Source: CAD feature listing. Evaluate the final solid. Frame: model axes, mm. Give positions to 0.01 mm unless a question says otherwise; leave off trailing zeros. Loops run counter-clockwise (first coordinate to the right, second up) from the corner with the lowest first, then second, coordinate; pieces in that order, holes last. Notation, with made-up numbers: M 11.25,-11 L 24.25,-11 A13 ccw 24.25,7 Z; hole C 16.5,61.25 d3. An arc over 180 degrees is marked long. Put each result on its own line as item: value.
Solid Edge part; units mm, degrees
sketch "Sketch1" plane through (0, 0, 0) normal (0, 0, 1) x (1, 0, 0)
  line L0 (4.0177, 12.988) -> (9.0177, 12.988)
  line L1 (59.0177, 12.988) -> (9.0177, 12.988)
  line L2 (64.0177, 12.988) -> (59.0177, 12.988)
  line L3 (64.0177, 7.988) -> (64.0177, 12.988)
  line L4 (64.0177, 2.988) -> (64.0177, 7.988)
  line L5 (59.0177, 2.988) -> (64.0177, 2.988)
  line L6 (9.0177, 2.988) -> (59.0177, 2.988)
  line L7 (4.0177, 2.988) -> (9.0177, 2.988)
  line L8 (4.0177, 7.988) -> (4.0177, 2.988)
  line L9 (4.0177, 7.988) -> (4.0177, 12.988)
extrude "Protrusion1" add sketch "Sketch1" along normal blind 4
fillet "Redondo_3" radius 5 4 edges at (64.0177, 2.988, 2) (64.0177, 12.988, 2) (4.0177, 2.988, 2) (4.0177, 12.988, 2)
hole "Furo_3" at (9.0177, 7.988, 4) direction (0, 0, -1) diameter 3 end up to next
hole "Hole1" at (59.0177, 7.988, 4) direction (0, 0, -1) diameter 3 end up to next
1. Contact query for flat-ended pins moving along their axis: P1, Ø2, axis at y = 6.5, z = 1, coming from the -X side; P2, Ø1.8, axis at x = 9.02, y = 7.99, coming from the +Z side; P3, Ø1, axis at y = 7, z = 1, coming from the +X side. Output: stop coordinate, or through.
Found:
P1: x = 4.04
P2: through
P3: x = 63.99
2. Section query B-B (z = 0.55). State how many separate pieces and enclosed holes the cut face has, plus the area to 3 significant figures.
Found:
separate pieces: 1
enclosed holes: 2
area: 564 mm^2
3. Draft query along Y for faces 1 (the cylindrical face through (62.5, 4.4, 2)), 2 (the flat face through (34, 8, 4)), 3 (the cylindrical face through (60.505, 8.183, 2.028)), 4 (the flat face through (34, 12.988, 2)). Return one class per face: pulls with the +Y half, pulls with the -Y half, needs draft (parallel to the pull), parting line crosses it, or undercut.
Found:
face 1: pulls with the -Y half
face 2: needs draft
face 3: undercut
face 4: pulls with the +Y half
4. Material intervals for line 1 (X direction, y = 9.25, z = 3.3); line 2 (X direction, y = 7.5, z = 3.85); line 3 (Y direction, x = 8, z = 2.9), sorted ascending. Write a range as from..to.
Found:
line 1: 4.18..8.21, 9.83..58.21, 59.83..63.86
line 2: 4.04..7.6, 10.44..57.6, 60.44..63.99
line 3: 3.09..6.89, 9.09..12.88
5. Section query A-A (y = 8.5). Output: boundary loops of the cut face in (x, z).
Found:
outline: M 4.04,0 L 7.61,0 L 7.61,4 L 4.04,4 Z; M 10.43,0 L 57.61,0 L 57.61,4 L 10.43,4 Z; M 60.43,0 L 63.99,0 L 63.99,4 L 60.43,4 Z
6. Section query D-D (y = 5). Output: boundary loops of the cut face in (x, z).
Found:
outline: M 5.01,0 L 63.03,0 L 63.03,4 L 5.01,4 Z
7. Section query C-C (y = 12). Output: boundary loops of the cut face in (x, z), plus the area to 3 significant figures.
Found:
outline: M 6.03,0 L 62,0 L 62,4 L 6.03,4 Z
area: 224 mm^2
